Could you check a few things on this model? Use its own coordinates, in mm. Give positions to 0.01 mm unless a question says otherwise; leave off trailing zeros. Loops run counter-clockwise (first coordinate to the right, second up) from the corner with the lowest first, then second, coordinate; pieces in that order, holes last. Notation, with made-up numbers: M 11.5,6.5 L 18.5,6.5 A23 cw 18.5,17.5 Z; hole C 88.5,33.5 d8. An arc over 180 degrees is marked long. Return JSON: item names as keys, results as strings. Group by question number.
1. If we section it at D-D (z = 30): Write out the boundary of the cut face in (x, y).
2. If we section it at B-B (x = 15): Write out the boundary of the cut face in (y, z).
3. If we section it at C-C (y = 14.45): Write out the boundary of the cut face in (x, z), plus the area to 4 significant figures.
4. For pin 1 (7.5 mm diameter, centred on x = 193, y = 45.45, fed in from -Z), with a flat end and sliding along its axis, tell me the tip position at first contact or that it passes through.
5. Please list where these lines run through material, in increasing order: line 1 (X direction, y = 45.45, z = 25.5); line 2 (Y direction, x = 39, z = 9); line 3 (X direction, y = 53.5, z = 9.5).
6. If we section it at A-A (y = 45.45): Write out the boundary of the cut face in (x, z).
```python
from build123d import *

# Parameters (mm, degrees)
F0_W     = 208
F0_H     = 57
F1_DEPTH = 35
F3_D     = 6.8
F3_DEPTH = 30
F3_TIP   = 2.0429261047
F4_D     = 8.5


with BuildPart() as f1:
    # F0 (on Top) → F1 (new body)
    with BuildSketch(Plane.XY):
        with Locations((104, 28.5)):
            Rectangle(F0_W, F0_H)
    extrude(amount=F1_DEPTH)

    # F3
    with Locations(Plane(origin=(0, 57, 0), x_dir=(-1, 0, 0), z_dir=(0, 1, 0))):
        with Locations((-9.5570590347, 9)):
            Hole(F3_D / 2, depth=F3_DEPTH)
            with Locations((0, 0, -(F3_DEPTH + F3_TIP / 2))):  # 118° drill point
                Cone(0, F3_D / 2, F3_TIP, mode=Mode.SUBTRACT)

    # F4 (through all)
    with Locations(Plane(origin=(0, 0, 0), x_dir=(1, 0, 0), z_dir=(0, 0, -1))):
        with Locations((193, -45.45), (169, -14.45), (39, -45.45), (15, -14.45)):
            Hole(F4_D / 2)


solid = f1.part
```
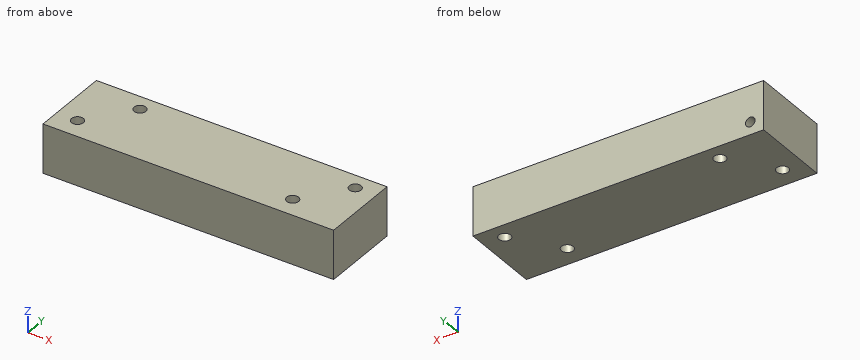
Answer:
{
 "1": {"outline": "M 0,0 L 208,0 L 208,57 L 0,57 Z; hole C 15,14.45 d8.5; hole C 39,45.45 d8.5; hole C 169,14.45 d8.5; hole C 193,45.45 d8.5"},
 "2": {"outline": "M 0,0 L 10.2,0 L 10.2,35 L 0,35 Z; M 18.7,0 L 57,0 L 57,35 L 18.7,35 Z"},
 "3": {"outline": "M 0,0 L 10.75,0 L 10.75,35 L 0,35 Z; M 19.25,0 L 164.75,0 L 164.75,35 L 19.25,35 Z; M 173.25,0 L 208,0 L 208,35 L 173.25,35 Z", "area": "6,685 mm²"},
 "4": {"pin 1": "passes through"},
 "5": {"line 1": "x = 0 to 34.75, 43.25 to 188.75, 197.25 to 208", "line 2": "y = 0 to 41.2, 49.7 to 57", "line 3": "x = 0 to 6.19, 12.92 to 208"},
 "6": {"outline": "M 0,0 L 34.75,0 L 34.75,35 L 0,35 Z; M 43.25,0 L 188.75,0 L 188.75,35 L 43.25,35 Z; M 197.25,0 L 208,0 L 208,35 L 197.25,35 Z; hole C 9.56,9 d6.8"}
}
